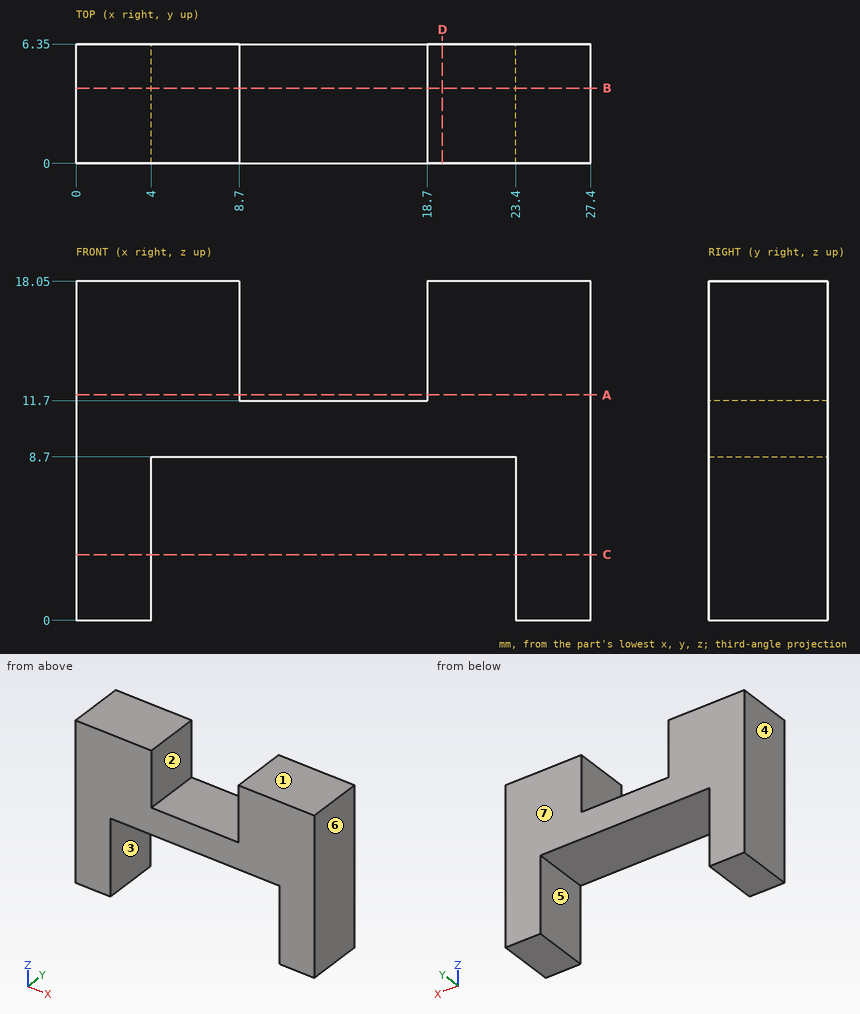
Verification items for this drawing (mm, ordinates from the low corner). A direction names the side the tool comes from. Coordinates: 2 decimals unless noted, no trailing zeros. Loops run counter-clockwise (first coordinate to the right, second up) from the corner with the lowest first, then second, coordinate; pieces in that order, holes last. Notation, with made-up numbers: (14.25, -27) -> (42.25, -27) arc R12 cw to (42.25, -19) -> close; hole circle Ø10 at (58.25, 31). An arc over 180 degrees is marked (long way). Answer in a Markdown table with one row per item. Add a question column.
1. Depth check by flat-ended pin: P1, Ø1.9, axis at x = 10, y = 2.5, coming from the -Z side. Enter the tip coordinate at first touch or a pass-through.
2. Material ranges on probe 1 along X at (y, z) = (3.25, 1.75); probe 2 along X at (y, z) = (4.75, 17); probe 3 along Z at (x, y) = (14.5, 5.5), recorded low to high. Write a range as [from, to].
3. Section check B-B, the plane y = 4. Enter the section's corners in (x, z), then the cut area to 3 significant figures.
4. Section check D-D, the plane x = 19.5. Enter the section's corners in (y, z), then the cut area to 3 significant figures.
5. Section check C-C, the plane z = 3.5. Enter the section's corners in (x, y), then the cut area to 3 significant figures.
6. Access from +Z, -Z, +X, -X, +Y, -Y to the whole of each face (thin tool, end or side, straight path). Record for the marked faces 1, 2 and 3.
7. Draft check along X on the marked faces 4, 5, 6 and 7. Enter one of: +X half, -X half, draft (parallel to the pull), parting line (faces both ways), or undercut.
8. Section check A-A, the plane z = 12. Enter the section's corners in (x, y).
Derived:
| question | item | result |
|---|---|---|
| 1 | P1 | stops at z = 8.7 |
| 2 | probe 1 | x = [0, 4], [23.4, 27.4] |
| 2 | probe 2 | x = [0, 8.7], [18.7, 27.4] |
| 2 | probe 3 | z = [8.7, 11.7] |
| 3 | outline | (0, 0) -> (4, 0) -> (4, 8.7) -> (23.4, 8.7) -> (23.4, 0) -> (27.4, 0) -> (27.4, 18.05) -> (18.7, 18.05) -> (18.7, 11.7) -> (8.7, 11.7) -> (8.7, 18.05) -> (0, 18.05) -> close |
| 3 | area | 262 mm² |
| 4 | outline | (0, 8.7) -> (6.35, 8.7) -> (6.35, 18.05) -> (0, 18.05) -> close |
| 4 | area | 59.4 mm² |
| 5 | outline | (0, 0) -> (4, 0) -> (4, 6.35) -> (0, 6.35) -> close; (23.4, 0) -> (27.4, 0) -> (27.4, 6.35) -> (23.4, 6.35) -> close |
| 5 | area | 50.8 mm² |
| 6 | face 1 | +Z, +X, -X, +Y, -Y |
| 6 | face 2 | +Z, +Y, -Y |
| 6 | face 3 | -Z, +Y, -Y |
| 7 | face 4 | -X half |
| 7 | face 5 | undercut |
| 7 | face 6 | +X half |
| 7 | face 7 | draft |
| 8 | outline | (0, 0) -> (8.7, 0) -> (8.7, 6.35) -> (0, 6.35) -> close; (18.7, 0) -> (27.4, 0) -> (27.4, 6.35) -> (18.7, 6.35) -> close |
